Part print with two shaded views. Sizes in mm from the minimum x, y, z corner. A direction names the side the tool comes from. Round coordinates to 2 decimals unless told otherwise and drop trailing zeros. Loops run counter-clockwise (first coordinate to the right, second up) from the corner with the lowest first, then second, coordinate; pieces in that order, holes last. Notation, with made-up numbers: (69.5, 17) - (107.5, 17) arc R19 cw to (107.5, 38) - close; hole circle Ø11 at (-18.5, 25.5). An arc over 180 degrees is marked (long way). Put each result on its own line as item: value. Start each with the question number.
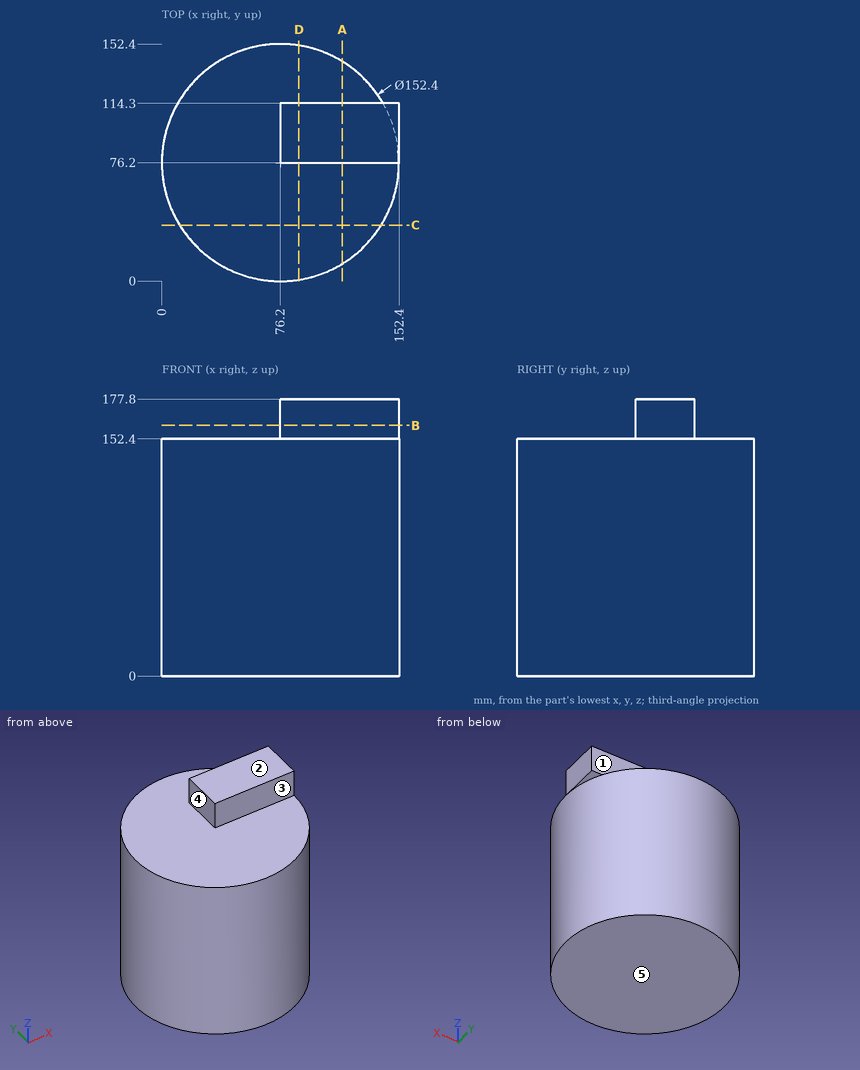
1) Slice it at B-B, the plane z = 161. Write the cut outline in (x, y).
2) Slice it at C-C, the plane y = 36. Write the cut outline in (x, z), and give its area (3 significant figures).
3) Drop flat-ended pins along their axis: pin 1 Ø7.5 at (x, z) = (117, 169.5) entering from -Y; pin 2 Ø10 at (x, z) = (58, 84.5) entering from -Y; pin 3 Ø8 at (y, z) = (41.5, 61) entering from -X. Give the stop position or say it passes through.
4) Slice it at D-D, the plane x = 88. Write the cut outline in (y, z), and give its area (3 significant figures).
5) Slice it at A-A, the plane x = 116. Write the cut outline in (y, z).
6) Which spindle directions (+Z, -Z, +X, -X, +Y, -Y) get a long thin tool onto all of the face, cutting with end or side? Do the marked faces 1, 2, 3, 4 and 5. Say none if no direction does.
7) Drill centre lines: line 1 (Z direction, x = 15.5, y = 34.5); line 2 (Y direction, x = 136, z = 156); line 3 (Y direction, x = 114, z = 90). Where is each one in solid material? Low to high. Write a range as [from, to].
Taken from the geometry:
1. outline: (76.2, 76.2) - (152.4, 76.2) - (152.4, 114.3) - (76.2, 114.3) - close
2. outline: (11.47, 0) - (140.93, 0) - (140.93, 152.4) - (11.47, 152.4) - close
2. area: 19,700 mm2
3. pin 1: stops at y = 76.2
3. pin 2: stops at y = 1.15
3. pin 3: stops at x = 6.46
4. outline: (0.92, 0) - (151.48, 0) - (151.48, 152.4) - (114.3, 152.4) - (114.3, 177.8) - (76.2, 177.8) - (76.2, 152.4) - (0.92, 152.4) - close
4. area: 23,900 mm2
5. outline: (11.22, 0) - (141.18, 0) - (141.18, 152.4) - (114.3, 152.4) - (114.3, 177.8) - (76.2, 177.8) - (76.2, 152.4) - (11.22, 152.4) - close
6. face 1: +Z, +X, -X, +Y
6. face 2: +Z, +X, -X, +Y, -Y
6. face 3: +Z, +X, -X, -Y
6. face 4: +Z, -X, +Y, -Y
6. face 5: -Z, +X, -X, +Y, -Y
7. line 1: z = [0, 152.4]
7. line 2: y = [76.2, 114.3]
7. line 3: y = [10.04, 142.36]
